Here's how the part is built. I have some questions about the finished solid (model axes, mm). Face numbers are marked on the shaded views. Coordinates: 2 decimals unless noted, no trailing zeros. Write each loop counter-clockwise with the first axis right and the second up, starting at its lowest first coordinate (ties: lowest second). Pieces come first, ordered by that corner, then holes. Notation, with made-up numbers: (70, -36) -> (94, -36) arc R17 ccw to (94, -27) -> close; hole circle Ø5 at (88, 85.25). An arc over 180 degrees is marked (long way). Put each result on its own line as item: value. Start each with the question number.
Item 1: I want a section at A-A, the plane z = 0. List the corners of the cut face in (x, y) for me (3 decimals), then the cut area to 3 significant figures.
Item 2: For pin 1 (5 mm diameter, centred on x = -22.5, z = -18.5, fed in from -Y); pin 2 (12 mm diameter, centred on y = 3.5, z = 23.5, fed in from +X); pin 3 (5 mm diameter, centred on x = 2, y = 7, fed in from -Z) (3 decimals); pin 4 (1.5 mm diameter, centred on x = 14.5, y = 12, fed in from +Z), each with a flat end and sliding along its axis, tell me the tip position at first contact or that it passes through.
Item 3: If we mould it in two halves opening along Z, with no side actions, what happens to the marked faces 1, 2 and 3? For each: released by +Z, released by -Z, zero draft, split by the parting line, or undercut.
Item 4: I want a section at C-C, the plane y = 31. List the corners of the cut face in (x, z) for me (3 decimals), then the cut area to 3 significant figures.
Item 5: I want a section at B-B, the plane x = 0. List the corners of the cut face in (y, z) for me (3 decimals).
Item 6: I need wall thicknesses on line 1 (Z direction, x = 0, y = 25.5) (3 decimals); line 2 (Y direction, x = -26.5, z = 8.5); line 3 (X direction, y = 6, z = 9). Which ranges of each line are inside material? Lowest first, please. Write a range as [from, to].
from build123d import *


with BuildPart() as part:
    # Sketch1 → Revolve1 (revolve)
    with BuildSketch(Plane.XY):
        with BuildLine():
            Line((22.125, 33.5), (22.125, 4))
            ThreePointArc((22.125, 4), (22.710786438, 2.585786438), (24.125, 2))
            Line((24.125, 2), (34.625, 2))
            ThreePointArc((34.625, 2), (34.978553391, 1.853553391), (35.125, 1.5))
            Line((35.125, 1.5), (35.125, 0))
            Line((35.125, 0), (20.125, 0))
            Line((20.125, 0), (20.125, 33.5))
            ThreePointArc((20.125, 33.5), (20.271446609, 33.853553391), (20.625, 34))
            Line((20.625, 34), (21.625, 34))
            ThreePointArc((21.625, 34), (21.978553391, 33.853553391), (22.125, 33.5))
        make_face()
    revolve(axis=Axis((0, 40.764727394, 0), (0, -1, 0)))


solid = part.part
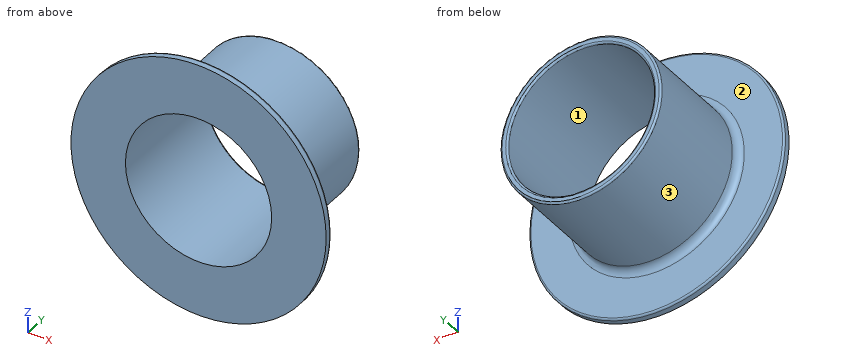
Calculated:
1. outline: (-35.125, 0) -> (-20.125, 0) -> (-20.125, 33.5) arc R0.5 ccw to (-20.625, 34) -> (-21.625, 34) arc R0.5 ccw to (-22.125, 33.5) -> (-22.125, 4) arc R2 cw to (-24.125, 2) -> (-34.625, 2) arc R0.5 ccw to (-35.125, 1.5) -> close; (20.125, 0) -> (35.125, 0) -> (35.125, 1.5) arc R0.5 ccw to (34.625, 2) -> (24.125, 2) arc R2 cw to (22.125, 4) -> (22.125, 33.5) arc R0.5 ccw to (21.625, 34) -> (20.625, 34) arc R0.5 ccw to (20.125, 33.5) -> close
1. area: 189 mm2
2. pin 1: stops at y = 0
2. pin 2: stops at x = 30.26
2. pin 3: stops at z = -22.125
2. pin 4: stops at z = 17.33
3. face 1: undercut
3. face 2: zero draft
3. face 3: split by the parting line
4. outline: circle Ø44.25 at (0, 0); hole circle Ø40.25 at (0, 0)
4. area: 265 mm2
5. outline: (0, -35.125) -> (1.5, -35.125) arc R0.5 ccw to (2, -34.625) -> (2, -24.125) arc R2 cw to (4, -22.125) -> (33.5, -22.125) arc R0.5 ccw to (34, -21.625) -> (34, -20.625) arc R0.5 ccw to (33.5, -20.125) -> (0, -20.125) -> close; (0, 20.125) -> (33.5, 20.125) arc R0.5 ccw to (34, 20.625) -> (34, 21.625) arc R0.5 ccw to (33.5, 22.125) -> (4, 22.125) arc R2 cw to (2, 24.125) -> (2, 34.625) arc R0.5 ccw to (1.5, 35.125) -> (0, 35.125) -> close
6. line 1: z = [-22.125, -20.125], [20.125, 22.125]
6. line 2: y = [0, 2]
6. line 3: x = [-20.21, -18], [18, 20.21]
